Verification items for the finished model (mm, model axes). A direction names the side the tool comes from. Coordinates: 2 decimals unless noted, no trailing zeros. Write each loop counter-clockwise with the first axis right and the second up, starting at its lowest first coordinate (ties: lowest second). Pieces come first, ordered by that corner, then holes. Notation, with made-up numbers: M 69.25,47.5 L 84.25,47.5 A10 ccw 84.25,61.5 Z; hole C 58,60 d9. An arc over 180 degrees is marked long. One line per item, written item: value.
Autodesk Inventor part; units mm, degrees
ref_plane "YZ Plane" through (0, 0, 0) normal (1, 0, 0) x (0, 1, 0)
ref_plane "XZ Plane" through (0, 0, 0) normal (0, 1, 0) x (-1, 0, 0)
ref_plane "XY Plane" through (0, 0, 0) normal (0, 0, 1) x (1, 0, 0)
sketch "Эскиз1" plane through (0, 0, 0) normal (0, 0, 1) x (1, 0, 0)
  line L0 (-49, 0) -> (49, 0)
  line L1 (-6.7712, 10) -> (6.7712, 10)
  line L2 (6.7712, -10) -> (-6.7712, -10)
  line L3 (0, -21) -> (0, 21)
  arc A0 (-10.0784, 11.25) -> (-10.0784, -11.25) centre (-20, 0) ccw
  arc A1 (10.0784, -11.25) -> (10.0784, 11.25) centre (20, 0) ccw
  circle A2 centre (-20, 0) radius 5
  circle A3 centre (20, 0) radius 5
  arc A4 (-10.0784, 11.25) -> (-6.7712, 10) centre (-6.7712, 15) ccw
  arc A5 (-6.7712, -10) -> (-10.0784, -11.25) centre (-6.7712, -15) ccw
  arc A6 (10.0784, -11.25) -> (6.7712, -10) centre (6.7712, -15) ccw
  arc A7 (6.7712, 10) -> (10.0784, 11.25) centre (6.7712, 15) ccw
  point P0 (0, 0)
  point P1 (-8.8197, 10)
  point P2 (8.8197, -10)
  point P3 (8.8197, 10)
  point P4 (-8.8197, -10)
  dimension "d1" = 20
  dimension "d3" = 15
  dimension "d4" = 10
  dimension "d5" = 5
  dimension "d8" = 40
extrude "Выдавливание1" add sketch "Эскиз1" along normal blind 10
sketch "Эскиз2" plane through (0, 0, 0) normal (0, 0, -1) x (-1, 0, 0)
  circle A0 centre (-20, 0) radius 5
  point P0 (0, 0)
extrude "Выдавливание2" cut sketch "Эскиз2" along normal through all both and the other way through all
sketch "Эскиз3" plane through (0, 0, 10) normal (0, 0, 1) x (1, 0, 0)
  circle A0 centre (-20, 0) radius 5
  point P0 (0, 0)
extrude "Выдавливание3" cut sketch "Эскиз3" along normal through all both and the other way through all
properties part number "кривошип_v1"
Item 1: Cross-section at D-D, the plane y = 4. Enter the section's corners in (x, z), and give its area (3 significant figures).
The answers:
outline: M -34.46,0 L -23,0 L -23,10 L -34.46,10 Z; M -17,0 L 17,0 L 17,10 L -17,10 Z; M 23,0 L 34.46,0 L 34.46,10 L 23,10 Z
area: 569 mm²
Item 2: Draft check along Y on faces 4 (the face through (8.56, 10.33, 4.93)), 5 (the face through (0, 0, 0)), 6 (the face through (-25, 0, 5)). Enter one of: released by +Y, released by -Y, zero draft, split by the parting line, or undercut.
The answers:
face 4: released by +Y
face 5: zero draft
face 6: undercut
Item 3: Go/stop test with flat-tipped pins: P1, Ø5, axis at y = 12, z = 5.5, coming from the +X side; P2, Ø3, axis at x = -2.5, z = 2.5, coming from the +Y side; P3, Ø5, axis at x = 2.5, z = 4.5, coming from the -Y side. Record where each tip stops, or that it passes through.
The answers:
P1: stops at x = 31.61
P2: stops at y = 10
P3: stops at y = -10
Item 4: Cross-section at C-C, the plane z = 8.5. Enter the section's corners in (x, y), and give its area (3 significant figures).
The answers:
outline: M -10.08,-11.25 A5 cw -6.77,-10 L 6.77,-10 A5 cw 10.08,-11.25 A15 ccw long 10.08,11.25 A5 cw 6.77,10 L -6.77,10 A5 cw -10.08,11.25 A15 ccw long Z; hole C -20,0 d10; hole C 20,0 d10
area: 1,510 mm²
Item 5: Scan lines: line 1 (Y direction, x = -20, z = 6); line 2 (X direction, y = -0.5, z = 9.25); line 3 (X direction, y = 4, z = 2.75). Record each from-to range of solid material in increasing order.
The answers:
line 1: y = -15 to -5, 5 to 15
line 2: x = -34.99 to -24.97, -15.03 to 15.03, 24.97 to 34.99
line 3: x = -34.46 to -23, -17 to 17, 23 to 34.46
Item 6: Access from +Z, -Z, +X, -X, +Y, -Y to the whole of each face (thin tool, end or side, straight path). Record for faces 1 (the face through (0, 10, 5)), 2 (the face through (0, 0, 10)), 3 (the face through (8.515, -10.314, 4.93)).
The answers:
face 1: +Z, -Z, +Y
face 2: +Z, +X, -X, +Y, -Y
face 3: +Z, -Z, -Y
Item 7: Cross-section at A-A, the plane y = 0. Enter the section's corners in (x, z), and give its area (3 significant figures).
The answers:
outline: M -35,0 L -25,0 L -25,10 L -35,10 Z; M -15,0 L 15,0 L 15,10 L -15,10 Z; M 25,0 L 35,0 L 35,10 L 25,10 Z
area: 500 mm²
Item 8: Cross-section at B-B, the plane x = -20. Enter the section's corners in (y, z).
The answers:
outline: M -15,0 L -5,0 L -5,10 L -15,10 Z; M 5,0 L 15,0 L 15,10 L 5,10 Z
